Part model, mm, in its own coordinate system. Face numbers are marked on the shaded views. A direction names the side the tool comes from. Give positions to 0.01 mm unless a question says otherwise; leave off trailing zeros. Write each loop counter-clockwise with the first axis right and the second up, starting at its lowest first coordinate (ties: lowest second). Pieces come first, ordered by that corner, then holes. Notation, with made-up numbers: M 69.25,-37 L 87.25,-37 A19 ccw 87.25,-10 Z; hole C 25,80 d6. An arc over 180 degrees is marked long. Use CSV: the item, a comma, the result in double quotes. Start each with the question number.
Item 1: Pin check, flat tips, straight feed: pin 1 (5 mm diameter, centred on y = -15, z = 10, fed in from +X); pin 2 (2 mm diameter, centred on y = -10, z = 24, fed in from -X); pin 3 (3 mm diameter, centred on x = 6.5, y = -19.5, fed in from -Z). Stop position of each tip, or through.
Item 2: Cut at A-A (x = 20.5). List the corners of the cut face in (y, z), then the cut area to 3 significant figures.
Item 3: Cut at C-C (z = 19). List the corners of the cut face in (x, y).
Item 4: Cut at B-B (y = -27.5). List the corners of the cut face in (x, z), then the cut area to 3 significant figures.
Item 5: Drill centre lines: line 1 (Y direction, x = 23.75, z = 9); line 2 (X direction, y = -11.5, z = 9); line 3 (X direction, y = -24.5, z = 8.5). Where is each one in solid material? Low to high. Write a range as [from, to].
Item 6: Cut at D-D (x = 7.25). List the corners of the cut face in (y, z).
Item 7: Which spindle directions (+Z, -Z, +X, -X, +Y, -Y) get a long thin tool onto all of the face, cutting with end or side? Do the marked faces 1, 2 and 3. Say none if no direction does.
Item 8: Mould opens along Y. For the marked faces 4, 5, 6 and 7 say: released by +Y, released by -Y, zero draft, split by the parting line, or undercut.
from build123d import *

# Parameters (mm, degrees)
F1_DEPTH = 30
F2_W     = 10
F2_H     = 10
F3_DEPTH = 30.001


with BuildPart() as f1:
    # F0 (on Front) → F1 (new body)
    with BuildSketch(Plane.XZ):
        Polygon((10, 10), (10, 0), (30, 0), (30, 10), (10, 30), (0, 30), (0, 10), align=None)
    extrude(amount=F1_DEPTH)

    # F2 (on face) → F3 (cut, through all)
    with BuildSketch(Plane(origin=(0, 0, 0), x_dir=(1, 0, 0), z_dir=(0, 0, -1))):
        with Locations((25, 15)):
            Rectangle(F2_W, F2_H)
    extrude(amount=-F3_DEPTH, mode=Mode.SUBTRACT)


solid = f1.part
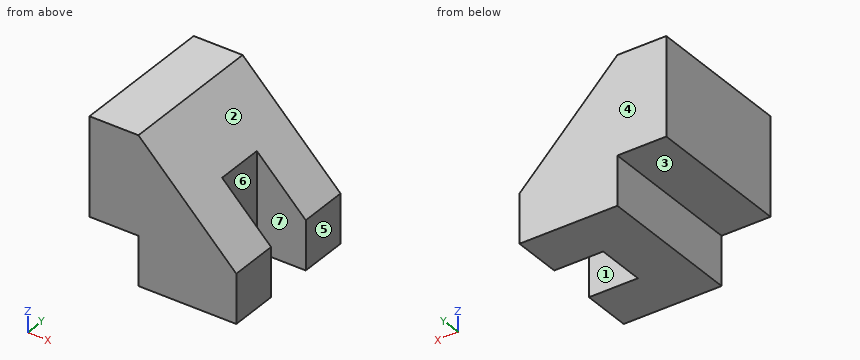
Worked answers:
1,pin 1,"stops at x = 20"
1,pin 2,"stops at x = 0"
1,pin 3,"stops at z = 10"
2,outline,"M -30,0 L -20,0 L -20,19.5 L -30,19.5 Z; M -10,0 L 0,0 L 0,19.5 L -10,19.5 Z"
2,area,"390 mm^2"
3,outline,"M 0,-30 L 21,-30 L 21,-20 L 20,-20 L 20,-10 L 21,-10 L 21,0 L 0,0 Z"
4,outline,"M 0,10 L 10,10 L 10,0 L 30,0 L 30,10 L 10,30 L 0,30 Z"
4,area,"600 mm^2"
5,line 1,"y = [-30, -20], [-10, 0]"
5,line 2,"x = [10, 20]"
5,line 3,"x = [10, 30]"
6,outline,"M -30,10 L 0,10 L 0,30 L -30,30 Z"
7,face 1,"+Z, -Z, +X"
7,face 2,"+Z, +X, +Y, -Y"
7,face 3,"-Z, -X, +Y, -Y"
8,face 4,"released by +Y"
8,face 5,"zero draft"
8,face 6,"undercut"
8,face 7,"undercut"
